Read the model definition and answer for the solid it produces. Units are mm, in the model's axes. A direction names the side the tool comes from. Give positions to 0.01 mm unless a question says otherwise; leave off trailing zeros. Order: outer loops, then holes, each group sorted by start corner. A loop starts at its lowest first (then second) coordinate and runs counter-clockwise, first axis right, second up. Notation, with made-up numbers: (13.5, 21.25) -> (61.5, 21.25) arc R21 cw to (61.5, 28.25) -> close; hole circle Ø6 at (88.25, -5.5). An arc over 180 degrees is marked (long way). Answer as CSV lines item,"result". Start each with the question number.
1) Find section D-D (x = 62.25). Determine the outline of the cut face in (y, z) (3 decimals).
2) Flat-ended cylindrical pins translate along their axes: pin 1 Ø2 at (x, z) = (59.5, 79.5) entering from -Y; pin 2 Ø1.4 at (y, z) = (-53.5, 78.5) entering from +X; pin 3 Ø2 at (x, y) = (62, -60.5) entering from +Z. Find the tip coordinate at first contact, or state that the pin passes through.
3) The mould has two halves that part along Z. Classify faces 1 (the face through (54.29, -53.56, 77.92)), 2 (the face through (63.25, -59, 80)), 3 (the face through (57.33, -57.9, 80.72)): +Z half, -Z half, draft (parallel to the pull), parting line (faces both ways), or undercut.
4) Find section B-B (x = 55). Determine the outline of the cut face in (y, z) (3 decimals).
5) Find section C-C (y = -56.75). Determine the outline of the cut face in (x, z).
6) Find section A-A (z = 78.5). Determine the outline of the cut face in (x, y), and give its area (3 significant figures).
7) For faces 4 (the face through (57.334, -58.541, 78.563)), 5 (the face through (60.208, -54.661, 78.825)), determine the directions among +Z, -Z, +X, -X, +Y, -Y from which every point of the face is accessible in a straight line to the end or side of a thin tool.
8) Straight lines are drawn through the part: L1, parallel to X at y = -52.25, z = 78.85; L2, parallel to Z at x = 58.5, y = -55.25; L3, parallel to Z at x = 61.5, y = -60. For each, find the intervals that lie inside material, in ascending order. Write a range as from..to.
```python
from build123d import *

# Parameters (mm, degrees)
SKETCH_1_R          = 0.625
EXTRUDE_1_DEPTH     = 12
CUT_EXTRUDE_START   = -6
SKETCH_2_R          = 1.375
CUT_EXTRUDE_1_DEPTH = 6
CUT_EXTRUDE_2_DEPTH = 6


with BuildPart() as part:
    # 草图1 → 凸台-拉伸1 (new body)
    with BuildSketch(Plane(origin=(63.25, 0, 0), x_dir=(0, 0, -1), z_dir=(1, 0, 0))):
        with BuildLine():
            Line((-79.908766601, -63.245730904), (-77.178061801, -53.70329142))
            ThreePointArc((-77.178061801, -53.70329142), (-78.188696573, -51.985703477), (-79.853262586, -53.081473056))
            Line((-79.853262586, -53.081473056), (-81.6111671, -62.850028308))
            ThreePointArc((-81.6111671, -62.850028308), (-80.948102181, -63.857279605), (-79.908766601, -63.245730904))
        make_face()
        with Locations((-78.5, -53.325)):
            Circle(SKETCH_1_R, mode=Mode.SUBTRACT)
    extrude(amount=-EXTRUDE_1_DEPTH)

    # 草图2 → 切除-拉伸1 (cut)
    with BuildSketch(Plane(origin=(63.25, 0, 0), x_dir=(0, 0, -1), z_dir=(1, 0, 0)).offset(CUT_EXTRUDE_START)):
        with Locations((-78.5, -53.325)):
            Circle(SKETCH_2_R)
    extrude(amount=CUT_EXTRUDE_1_DEPTH, mode=Mode.SUBTRACT)

    # 草图3 → 切除-拉伸2 (cut)
    with BuildSketch(Plane(origin=(63.25, 0, 0), x_dir=(0, 0, -1), z_dir=(1, 0, 0)).offset(CUT_EXTRUDE_START)):
        with BuildLine():
            Line((-79.853262586, -53.081473056), (-80.060943062, -54.235539267))
            ThreePointArc((-80.060943062, -54.235539267), (-79.870673692, -54.036118774), (-79.612603732, -54.132921987))
            ThreePointArc((-79.612603732, -54.132921987), (-79.840339654, -53.631781049), (-79.853262586, -53.081473056))
        make_face()
        with BuildLine():
            ThreePointArc((-77.178061801, -53.70329142), (-77.432371823, -54.191484319), (-77.857788029, -54.540807873))
            ThreePointArc((-77.857788029, -54.540807873), (-77.583479618, -54.567749621), (-77.500669801, -54.83064408))
            Line((-77.500669801, -54.83064408), (-77.178061801, -53.70329142))
        make_face()
    extrude(amount=CUT_EXTRUDE_2_DEPTH, mode=Mode.SUBTRACT)


solid = part.part
```
Findings below:
1,outline,"(-63.246, 79.909) -> (-54.831, 77.501) arc R0.25 ccw to (-54.541, 77.858) arc R1.375 cw to (-54.133, 79.613) arc R0.25 ccw to (-54.236, 80.061) -> (-62.85, 81.611) arc R0.875 ccw to start"
2,pin 1,"y = -63.84"
2,pin 2,"x = 57.25"
2,pin 3,"z = 81.37"
3,face 1,"undercut"
3,face 2,"draft"
3,face 3,"+Z half"
4,outline,"(-63.246, 79.909) -> (-53.703, 77.178) arc R1.375 ccw (long way) to (-53.081, 79.853) -> (-62.85, 81.611) arc R0.875 ccw to start; hole circle Ø1.25 at (-53.325, 78.5)"
5,outline,"(51.25, 78.05) -> (63.25, 78.05) -> (63.25, 80.51) -> (51.25, 80.51) -> close"
6,outline,"(51.25, -58.32) -> (63.25, -58.32) -> (63.25, -54.7) -> (57.25, -54.7) -> (57.25, -53.95) -> (51.25, -53.95) -> close; (51.25, -52.7) -> (57.25, -52.7) -> (57.25, -51.95) -> (51.25, -51.95) -> close"
6,area,"52.5 mm²"
7,face 4,"-Z, +X, -X, -Y"
7,face 5,"+X, +Y"
8,L1,"51.25..57.25"
8,L2,"77.62..80.24"
8,L3,"78.98..81.1"
